Could you check a few things on this model? Use its own coordinates, in mm. A direction names the side the tool comes from. Round coordinates to 2 decimals unless told otherwise and drop trailing zeros. Order: outer loops, then holes, each group sorted by start corner. A loop starts at its lowest first (then second) coordinate and runs counter-clockwise, first axis right, second up. Notation, with made-up numbers: M -28,77 L -16,77 A16 ccw -16,97 Z; hole C -23.5,7.25 d2. An arc over 180 degrees is marked long. Write each question's results on one line, items separated by ' | '. Start each with the question number.
1. Suppose I cut it at D-D on z = -4. Write out the boundary of the cut face in (x, y) (3 decimals), and give its area (3 significant figures).
2. Suppose I cut it at A-A on x = 29.5. Write out the boundary of the cut face in (y, z) (3 decimals).
3. I'm going to push flat-ended pins straight in: pin 1 (1.5 mm diameter, centred on x = 24.5, z = -1, fed in from +Y); pin 2 (1.6 mm diameter, centred on x = 21, y = 2, fed in from -Z). Where does each tip first touch, or does it pass through?
4. For faces 5 (the flat face through (11, 3.175, 0)), 6 (the flat face through (22, 2, -4.5)), 7 (the flat face through (33, 2, 0)), which set-ups out of +Z, -Z, +X, -X, +Y, -Y let a thin tool reach every point of the face, with its end or its side?
5. Please list where these lines run through material, in increasing order: L1, parallel to X at y = 0.2, z = 0 (3 decimals); L2, parallel to Z at x = 30, y = 1 (3 decimals); L3, parallel to Z at x = 0, y = 0.15 (3 decimals).
6. Suppose I cut it at C-C on x = 7. Write out the boundary of the cut face in (y, z) (3 decimals), and give its area (3 significant figures).
7. We'd pull the mould along Z, two halves only. Please class faces 1 (the flat face through (25, 2, 3.175)), 2 (the flat face through (22, 2, 4.5)), 3 (the flat face through (25, 2, -3.175)), 4 (the cylindrical face through (-7.495, 1.565, 0.262)): released by +Z, released by -Z, zero draft, split by the parting line, or undercut.
8. Suppose I cut it at B-B on y = 2.45. Give the number of separate pieces and of enclosed holes in the cut face, and give its area (3 significant figures).
from build123d import *

# Parameters (mm, degrees)
SKETCH1_R             = 2
SKETCH1_W             = 16
SKETCH1_H             = 6.35
BOSS_EXTRUDE1_DEPTH   = 3.175
INDENT2_START         = 0.275
INDENT2_OUTLINE_R     = 2
INDENT2_DEPTH         = 2.9
INDENT2_2_OUTLINE_R   = 2.075
INDENT2_2_OUTLINE_R_2 = 2
INDENT2_2_DEPTH       = 0.275
FILLET4_R             = 0.05


# Read off the part's stored shape, not the designer's step: Indent2
with BuildPart() as part:
    # Sketch1 → Boss-Extrude1 (new body)
    with BuildSketch(Plane(origin=(0, 0, 0), x_dir=(1, 0, 0), z_dir=(0, 1, 0))):
        with BuildLine():
            Line((6, 4.5), (38, 4.5))
            Line((38, 4.5), (38, -4.5))
            Line((38, -4.5), (6, -4.5))
            ThreePointArc((6, -4.5), (-7.5, 0), (6, 4.5))
        make_face()
        with Locations(Location((0, 0, 0), (0, 0, 270))):
            Circle(SKETCH1_R, mode=Mode.SUBTRACT)
        with Locations((25, 0)):
            Rectangle(SKETCH1_W, SKETCH1_H, mode=Mode.SUBTRACT)
    extrude(amount=BOSS_EXTRUDE1_DEPTH)

    # Indent2 outline → Indent2 (cut)
    with BuildSketch(Plane(origin=(0, 0, 0), x_dir=(1, 0, 0), z_dir=(0, 1, 0)).offset(INDENT2_START)):
        with BuildLine():
            Line((1.973202198, -0.621873827), (2.310555802, -0.549506038))
            ThreePointArc((2.310555802, -0.549506038), (2.348957068, -0.350750187), (2.370293408, -0.149446173))
            Line((2.370293408, -0.149446173), (2.068796389, 0.018315857))
            Line((2.068796389, 0.018315857), (2.367275856, 0.191389711))
            ThreePointArc((2.367275856, 0.191389711), (2.342378694, 0.392284402), (2.300464399, 0.590329188))
            Line((2.300464399, 0.590329188), (1.961882375, 0.656712657))
            Line((1.961882375, 0.656712657), (2.192270455, 0.913550902))
            ThreePointArc((2.192270455, 0.913550902), (2.106511974, 1.096919461), (2.005449906, 1.272319015))
            Line((2.005449906, 1.272319015), (1.662925646, 1.230825847))
            Line((1.662925646, 1.230825847), (1.802670348, 1.546287365))
            ThreePointArc((1.802670348, 1.546287365), (1.664445185, 1.6941804), (1.514128003, 1.829765392))
            Line((1.514128003, 1.829765392), (1.201190168, 1.684457227))
            Line((1.201190168, 1.684457227), (1.236612307, 2.027662448))
            ThreePointArc((1.236612307, 2.027662448), (1.059450904, 2.125603157), (0.874592702, 2.208101584))
            Line((0.874592702, 2.208101584), (0.621873827, 1.973202197))
            Line((0.621873827, 1.973202197), (0.549506038, 2.310555802))
            ThreePointArc((0.549506038, 2.310555802), (0.350750187, 2.348957068), (0.149446173, 2.370293408))
            Line((0.149446173, 2.370293408), (-0.018315857, 2.068796389))
            Line((-0.018315857, 2.068796389), (-0.191389711, 2.367275856))
            ThreePointArc((-0.191389711, 2.367275856), (-0.392284402, 2.342378694), (-0.590329188, 2.300464399))
            Line((-0.590329188, 2.300464399), (-0.656712657, 1.961882375))
            Line((-0.656712657, 1.961882375), (-0.913550902, 2.192270455))
            ThreePointArc((-0.913550902, 2.192270455), (-1.096919461, 2.106511974), (-1.272319015, 2.005449905))
            Line((-1.272319015, 2.005449905), (-1.230825847, 1.662925646))
            Line((-1.230825847, 1.662925646), (-1.546287365, 1.802670348))
            ThreePointArc((-1.546287365, 1.802670348), (-1.6941804, 1.664445185), (-1.829765392, 1.514128003))
            Line((-1.829765392, 1.514128003), (-1.684457227, 1.201190168))
            Line((-1.684457227, 1.201190168), (-2.027662448, 1.236612307))
            ThreePointArc((-2.027662448, 1.236612307), (-2.125603157, 1.059450904), (-2.208101584, 0.874592702))
            Line((-2.208101584, 0.874592702), (-1.973202197, 0.621873827))
            Line((-1.973202197, 0.621873827), (-2.310555802, 0.549506038))
            ThreePointArc((-2.310555802, 0.549506038), (-2.348957068, 0.350750187), (-2.370293408, 0.149446173))
            Line((-2.370293408, 0.149446173), (-2.068796389, -0.018315857))
            Line((-2.068796389, -0.018315857), (-2.367275856, -0.191389711))
            ThreePointArc((-2.367275856, -0.191389711), (-2.342378694, -0.392284402), (-2.300464399, -0.590329188))
            Line((-2.300464399, -0.590329188), (-1.961882375, -0.656712657))
            Line((-1.961882375, -0.656712657), (-2.192270455, -0.913550902))
            ThreePointArc((-2.192270455, -0.913550902), (-2.106511974, -1.096919461), (-2.005449905, -1.272319015))
            Line((-2.005449905, -1.272319015), (-1.662925646, -1.230825847))
            Line((-1.662925646, -1.230825847), (-1.802670348, -1.546287365))
            ThreePointArc((-1.802670348, -1.546287365), (-1.664445185, -1.6941804), (-1.514128003, -1.829765392))
            Line((-1.514128003, -1.829765392), (-1.201190168, -1.684457227))
            Line((-1.201190168, -1.684457227), (-1.236612307, -2.027662448))
            ThreePointArc((-1.236612307, -2.027662448), (-1.059450904, -2.125603157), (-0.874592702, -2.208101584))
            Line((-0.874592702, -2.208101584), (-0.621873827, -1.973202198))
            Line((-0.621873827, -1.973202198), (-0.549506038, -2.310555802))
            ThreePointArc((-0.549506038, -2.310555802), (-0.350750187, -2.348957068), (-0.149446173, -2.370293408))
            Line((-0.149446173, -2.370293408), (0.018315857, -2.068796389))
            Line((0.018315857, -2.068796389), (0.191389711, -2.367275856))
            ThreePointArc((0.191389711, -2.367275856), (0.392284402, -2.342378694), (0.590329188, -2.300464399))
            Line((0.590329188, -2.300464399), (0.656712657, -1.961882375))
            Line((0.656712657, -1.961882375), (0.913550902, -2.192270455))
            ThreePointArc((0.913550902, -2.192270455), (1.096919461, -2.106511974), (1.272319015, -2.005449906))
            Line((1.272319015, -2.005449906), (1.230825847, -1.662925646))
            Line((1.230825847, -1.662925646), (1.546287365, -1.802670348))
            ThreePointArc((1.546287365, -1.802670348), (1.6941804, -1.664445185), (1.829765392, -1.514128003))
            Line((1.829765392, -1.514128003), (1.684457227, -1.201190168))
            Line((1.684457227, -1.201190168), (2.027662448, -1.236612307))
            ThreePointArc((2.027662448, -1.236612307), (2.125603157, -1.059450904), (2.208101584, -0.874592702))
            Line((2.208101584, -0.874592702), (1.973202198, -0.621873827))
        make_face()
        Circle(INDENT2_OUTLINE_R, mode=Mode.SUBTRACT)
    extrude(amount=INDENT2_DEPTH, mode=Mode.SUBTRACT)

    # Indent2 2 outline → Indent2 2 (cut)
    with BuildSketch(Plane(origin=(0, 0, 0), x_dir=(1, 0, 0), z_dir=(0, 1, 0))):
        Circle(INDENT2_2_OUTLINE_R)
        Circle(INDENT2_2_OUTLINE_R_2, mode=Mode.SUBTRACT)
    extrude(amount=INDENT2_2_DEPTH, mode=Mode.SUBTRACT)

    # Fillet4
    # the kernel refuses this fillet: 0.05 mm, written as the material it takes off along each edge
    with BuildSketch(Plane(origin=(2.068796389, 0.275, -0.018315857), x_dir=(0.8650868282896619, 0, -0.501622148155096), z_dir=(0, 1, 0)), Plane(origin=(1.961882375, 0.275, -0.656712657), x_dir=(0.6677366959947866, 0, -0.7443975448790559), z_dir=(0, 1, 0)), Plane(origin=(0.621873827, 0.275, -1.973202197), x_dir=(-0.20974448107145283, 0, -0.9777562337618038), z_dir=(0, 1, 0)), Plane(origin=(-0.018315857, 0.275, -2.068796389), x_dir=(-0.501622148155096, 0, -0.8650868282896619), z_dir=(0, 1, 0)), Plane(origin=(-0.656712657, 0.275, -1.961882375), x_dir=(-0.7443975448790559, 0, -0.6677366959947866), z_dir=(0, 1, 0)), Plane(origin=(-1.973202197, 0.275, -0.621873827), x_dir=(-0.9777562337618038, 0, 0.20974448107145283), z_dir=(0, 1, 0)), Plane(origin=(-2.068796389, 0.275, 0.018315857), x_dir=(-0.8650868282896619, 0, 0.501622148155096), z_dir=(0, 1, 0)), Plane(origin=(-1.961882375, 0.275, 0.656712657), x_dir=(-0.6677366959947866, 0, 0.7443975448790559), z_dir=(0, 1, 0)), Plane(origin=(0.018315857, 0.275, 2.068796389), x_dir=(0.501622148155096, 0, 0.8650868282896619), z_dir=(0, 1, 0)), Plane(origin=(0.656712657, 0.275, 1.961882375), x_dir=(0.7443975448790559, 0, 0.6677366959947866), z_dir=(0, 1, 0))) as fillet4_piece_1:
        with BuildLine():
            CenterArc((FILLET4_R * 1.76030903483, -FILLET4_R), FILLET4_R, 90, 120.799739684)
            Line((FILLET4_R * 0.901346811508, -FILLET4_R * 1.51203896229), (0, 0))
            Line((0, 0), (FILLET4_R * 1.76030903483, 0))
        make_face()
    extrude(amount=3.120038629, mode=Mode.SUBTRACT)
    with BuildSketch(Plane(origin=(1.662925646, 0.275, -1.230825847), x_dir=(0.40502384395389723, 0, -0.9143061226027139), z_dir=(0, 1, 0)), Plane(origin=(-1.230825847, 0.275, -1.662925646), x_dir=(-0.9143061226027142, 0, -0.40502384395389696), z_dir=(0, 1, 0)), Plane(origin=(-1.662925646, 0.275, 1.230825847), x_dir=(-0.40502384395389696, 0, 0.9143061226027142), z_dir=(0, 1, 0)), Plane(origin=(-0.621873827, 0.275, 1.973202198), x_dir=(0.20974448166583565, 0, 0.977756233634299), z_dir=(0, 1, 0)), Plane(origin=(1.230825847, 0.275, 1.662925646), x_dir=(0.9143061226027139, 0, 0.40502384395389723), z_dir=(0, 1, 0)), Plane(origin=(1.973202198, 0.275, 0.621873827), x_dir=(0.977756233634299, 0, -0.20974448166583565), z_dir=(0, 1, 0))) as fillet4_piece_2:
        with BuildLine():
            CenterArc((FILLET4_R * 1.76030903185, -FILLET4_R), FILLET4_R, 90, 120.799739601)
            Line((FILLET4_R * 0.901346807787, -FILLET4_R * 1.51203896104), (0, 0))
            Line((0, 0), (FILLET4_R * 1.76030903185, 0))
        make_face()
    extrude(amount=3.120038629, mode=Mode.SUBTRACT)
    with BuildSketch(Plane(origin=(1.201190168, 0.275, -1.684457227), x_dir=(0.10266443492130879, 0, -0.9947160468205429), z_dir=(0, 1, 0)), Plane(origin=(-1.684457227, 0.275, -1.201190168), x_dir=(-0.9947160468205429, 0, -0.10266443492130879), z_dir=(0, 1, 0)), Plane(origin=(-1.201190168, 0.275, 1.684457227), x_dir=(-0.10266443492130879, 0, 0.9947160468205429), z_dir=(0, 1, 0)), Plane(origin=(1.684457227, 0.275, 1.201190168), x_dir=(0.9947160468205429, 0, 0.10266443492130879), z_dir=(0, 1, 0))) as fillet4_piece_3:
        with BuildLine():
            CenterArc((FILLET4_R * 1.7603090297, -FILLET4_R), FILLET4_R, 90, 120.799739541)
            Line((FILLET4_R * 0.901346805096, -FILLET4_R * 1.51203896014), (0, 0))
            Line((0, 0), (FILLET4_R * 1.7603090297, 0))
        make_face()
    extrude(amount=3.120038629, mode=Mode.SUBTRACT)


solid = part.part
Filled sheet:
1) outline: M -6.344,0 L 38,0 L 38,3.175 L -6.344,3.175 Z | area: 141 mm^2
2) outline: M 0,-4.5 L 3.175,-4.5 L 3.175,-3.175 L 0,-3.175 Z; M 0,3.175 L 3.175,3.175 L 3.175,4.5 L 0,4.5 Z
3) pin 1: passes through | pin 2: stops at z = -4.5
4) face 5: +Z, -Z, +X, -X, +Y | face 6: -Z, +X, +Y, -Y | face 7: +Y, -Y
5) L1: x = -7.5 to -2.075, 2.075 to 17, 33 to 38 | L2: z = -4.5 to -3.175, 3.175 to 4.5 | L3: z = -7.5 to -2.075, 2.075 to 7.5
6) outline: M 0,-4.5 L 3.175,-4.5 L 3.175,4.5 L 0,4.5 Z | area: 28.6 mm^2
7) face 1: undercut | face 2: released by +Z | face 3: undercut | face 4: split by the parting line
8) separate pieces: 1 | enclosed holes: 2 | area: 337 mm^2
